```python
from build123d import *

# Parameters (mm, degrees)
SKETCH_1_R          = 25
EXTRUDE_1_DEPTH     = 5
SKETCH_2_R          = 18.525
CUT_EXTRUDE_1_DEPTH = 2
SKETCH_3_R          = 17
CUT_EXTRUDE_2_DEPTH = 3
SKETCH_4_R          = 2.1
CUT_EXTRUDE_3_DEPTH = 5


with BuildPart() as part:
    # ｽｹｯﾁ1 → ﾎﾞｽ - 押し出し1 (new body)
    with BuildSketch(Plane.XY):
        Circle(SKETCH_1_R)
    extrude(amount=EXTRUDE_1_DEPTH)

    # ｽｹｯﾁ2 → ｶｯﾄ - 押し出し1 (cut)
    with BuildSketch(Plane.XY.offset(5)):
        Circle(SKETCH_2_R)
    extrude(amount=-CUT_EXTRUDE_1_DEPTH, mode=Mode.SUBTRACT)

    # ｽｹｯﾁ3 → ｶｯﾄ - 押し出し2 (cut)
    with BuildSketch(Plane.XY.offset(3)):
        Circle(SKETCH_3_R)
    extrude(amount=-CUT_EXTRUDE_2_DEPTH, mode=Mode.SUBTRACT)

    # ｽｹｯﾁ4 → ｶｯﾄ - 押し出し3 (cut)
    with BuildSketch(Plane.XY.offset(5)):
        with Locations((15.379572491, 15.379572491)):
            Circle(SKETCH_4_R)
        with Locations((15.379572491, -15.379572491)):
            Circle(SKETCH_4_R)
        with Locations((-15.379572491, -15.379572491)):
            Circle(SKETCH_4_R)
        with Locations((-15.379572491, 15.379572491)):
            Circle(SKETCH_4_R)
    extrude(amount=-CUT_EXTRUDE_3_DEPTH, mode=Mode.SUBTRACT)


solid = part.part
```
The listing builds one solid part. Answer for the finished solid, in the listing's coordinates (mm). A direction names the side the tool comes from. Round coordinates to 2 decimals unless told otherwise and drop trailing zeros. Loops run counter-clockwise (first coordinate to the right, second up) from the corner with the lowest first, then second, coordinate; pieces in that order, holes last.
Q1. For a pull along Y with two mould halves and no side action, classify faces 3 (the face through (9.139, 14.334, 1.521)), 4 (the face through (3.6, -18.4, 5)), 5 (the face through (23.846, 7.509, 2.465)) as released by +Y, released by -Y, zero draft, split by the parting line, or undercut.
Q2. Find the intervals of material crossed by line 1 (Y direction, x = 14, z = 3.4); line 2 (X direction, y = 15, z = 4.5); line 3 (X direction, y = -15.5, z = 3.45), in increasing order.
Q3. Section D-D, the plane z = 2.1 is taken. Determine the outline of the cut face in (x, y), then the cut area to 3 significant figures.
Q4. Given pin 1 Ø3 at (x, z) = (-10, 2) entering from -Y; pin 2 Ø1 at (x, z) = (12.5, 4.5) entering from -Y; pin 3 Ø2 at (y, z) = (-2, 4) entering from -X; pin 4 Ø4 at (x, y) = (-15.38, -15.38) entering from -Z, each flat-ended and moving along its own axis, determine where each tip first touches the part or whether it passes through.
Q5. Which of the six approach directions +Z, -Z, +X, -X, +Y, -Y give full straight-line access (tool end or side, diameter ignored) to faces 1 (the face through (17.11, -7.1, 4.01)), 2 (the face through (17.32, 14.58, 2.54))?
Q6. Section C-C, the plane y = -16 is taken. Determine the outline of the cut face in (x, z).
Q7. Section A-A, the plane y = 0 is taken. Determine the outline of the cut face in (x, z) (3 decimals).
Completed:
1. face 3: undercut
1. face 4: zero draft
1. face 5: split by the parting line
2. line 1: y = -20.71 to -16.96, -13.8 to -12.13, 12.13 to 13.8, 16.96 to 20.71
2. line 2: x = -20 to -17.44, -13.31 to -10.87, 10.87 to 13.31, 17.44 to 20
2. line 3: x = -19.62 to -17.48, -13.28 to -10.15, 10.15 to 13.28, 17.48 to 19.62
3. outline: circle Ø50 at (0, 0); hole circle Ø4.2 at (-15.38, -15.38); hole circle Ø4.2 at (-15.38, 15.38); hole circle Ø34 at (0, 0); hole circle Ø4.2 at (15.38, -15.38); hole circle Ø4.2 at (15.38, 15.38)
3. area: 1,000 mm2
4. pin 1: stops at y = -23.51
4. pin 2: stops at y = -21.93
4. pin 3: stops at x = -24.98
4. pin 4: passes through
5. face 1: +Z
5. face 2: +Z, -Z
6. outline: (-19.21, 0) - (-17.39, 0) - (-17.39, 5) - (-19.21, 5) - close; (-13.37, 0) - (-5.74, 0) - (-5.74, 3) - (-9.34, 3) - (-9.34, 5) - (-13.37, 5) - close; (5.74, 0) - (13.37, 0) - (13.37, 5) - (9.34, 5) - (9.34, 3) - (5.74, 3) - close; (17.39, 0) - (19.21, 0) - (19.21, 5) - (17.39, 5) - close
7. outline: (-25, 0) - (-17, 0) - (-17, 3) - (-18.525, 3) - (-18.525, 5) - (-25, 5) - close; (17, 0) - (25, 0) - (25, 5) - (18.525, 5) - (18.525, 3) - (17, 3) - close
